Autodesk Inventor part; units mm, degrees
ref_plane "YZ Plane" through (0, 0, 0) normal (1, 0, 0) x (0, 1, 0)
ref_plane "XZ Plane" through (0, 0, 0) normal (0, 1, 0) x (-1, 0, 0)
ref_plane "XY Plane" through (0, 0, 0) normal (0, 0, 1) x (1, 0, 0)
sketch "스케치1" plane through (0, 0, 0) normal (0, 0, 1) x (1, 0, 0)
  line L0 (50, 0) -> (50, 28)
  line L1 (-50, 28) -> (-50, 0)
  line L2 (32, 28) -> (32, 38)
  line L3 (-32, 38) -> (-32, 28)
  line L4 (-40, 38) -> (-40, 60)
  line L5 (40, 60) -> (40, 38)
  line L6 (-35.94, 60) -> (-3.94, 28)
  line L7 (3.94, 28) -> (35.94, 60)
  line L8 (-40, 60) -> (-35.94, 60)
  line L9 (35.94, 60) -> (40, 60)
  line L10 (3.94, 28) -> (4.06, 28)
  line L11 (4.06, 28) -> (4.06, 24.06)
  line L12 (4.06, 24.06) -> (-3.94, 24.06)
  line L13 (-3.94, 24.06) -> (-3.94, 28)
  line L14 (-32, 28) -> (-3.94, 28)
  line L15 (3.94, 28) -> (32, 28)
  line L16 (50, 28) -> (3.94, 28)
  line L17 (-3.94, 28) -> (-50, 28)
  line L18 (32, 38) -> (13.94, 38)
  line L19 (-13.94, 38) -> (-32, 38)
  line L20 (40, 38) -> (13.94, 38)
  line L21 (-13.94, 38) -> (-40, 38)
  line L22 (4.06, 0) -> (5, 0)
  line L23 (5, 0) -> (5, 5.8283)
  line L24 (5, 5.8283) -> (-5, 5.8283)
  line L25 (-5, 5.8283) -> (-5, 0)
  line L26 (-50, 0) -> (-5, 0)
  line L27 (5, 0) -> (50, 0)
  point P0 (0, 0)
  point P1 (0, 0)
  dimension "d0" = 100
  dimension "d1" = 28
  dimension "d2" = 50
  dimension "d3" = 64
  dimension "d4" = 32
  dimension "d5" = 10
  dimension "d6" = 80
  dimension "d8" = 40
  dimension "d11" = 90
  dimension "d12" = 80
  dimension "d13" = 4.06
  dimension "d14" = 4.06
  dimension "d15" = 8
  dimension "d16" = 10
  dimension "d17" = 5
extrude "돌출1" add sketch "스케치1" along normal mid plane 48
sketch "스케치2" plane through (50, 0, 24) normal (1, 0, 0) x (0, 0, -1)
  line L0 (48, 0) -> (0, 0)
  line L1 (48, 5.8283) -> (0, 5.8283)
  line L2 (19.5, 0) -> (28.5, 0)
  line L3 (28.5, 0) -> (28.5, 5.8283)
  line L4 (28.5, 5.8283) -> (19.5, 5.8283)
  line L5 (19.5, 5.8283) -> (19.5, 0)
  point P0 (24, 0)
  dimension "d20" = 9
  dimension "d21" = 4.5
extrude "돌출2" cut sketch "스케치2" against normal through all
sketch "스케치3" plane through (-5, 5.8283, 24) normal (0, -1, 0) x (1, 0, 0)
  circle A0 centre (5, -24) radius 4.5
  dimension "d24" = 9
extrude "돌출3" cut sketch "스케치3" against normal through all
properties part number "부품1"
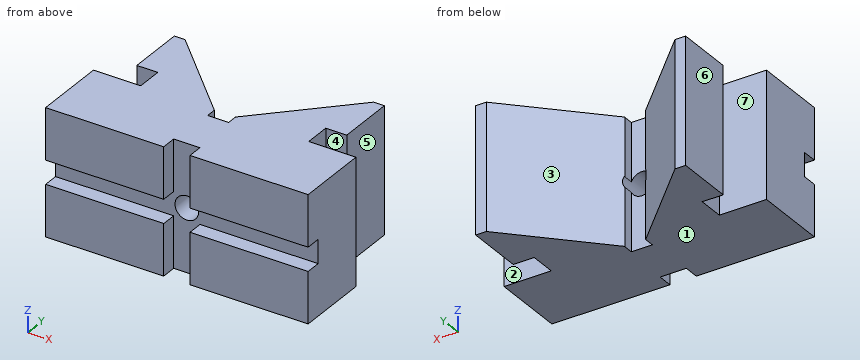
Here's how the part is built. I have some questions about the finished solid (model axes, mm). Face numbers are marked on the shaded views. A direction names the side the tool comes from. Round coordinates to 2 decimals unless told otherwise and drop trailing zeros. Write each loop counter-clockwise with the first axis right and the second up, starting at its lowest first coordinate (ties: lowest second). Pieces come first, ordered by that corner, then holes.
Q1. Which directions (+Z, -Z, +X, -X, +Y, -Y) give clear straight access to the entire face, cutting with the end or side of a thin tool? Please do the marked faces 5, 6 and 7.
Q2. Will these pins go through, and if not, where does the flat tip stop? P1, Ø11.5, axis at x = 0, z = 0, coming from the -Y side; P2, Ø6, axis at x = -13.5, z = 18, coming from the +Y side; P3, Ø5, axis at y = 34.5, z = -5.5, coming from the -X side.
Q3. If we section it at B-B on z = 0: Write out the boundary of the cut face in (x, y), plus the area to 3 significant figures.
Q4. Please list where these lines run through material, in increasing order: probe 1 along X at (y, z) = (21, 0); probe 2 along Z at (x, y) = (0, 11.5); probe 3 along X at (y, z) = (4.5, 21).
Q5. If we section it at A-A on y = 48: Write out the boundary of the cut face in (x, z), plus the area to 3 significant figures.
Q6. If we section it at C-C on x = -34: Write out the boundary of the cut face in (y, z), plus the area to 3 significant figures.
Q7. If we section it at D-D on x = 17.5: Write out the boundary of the cut face in (y, z), plus the area to 3 significant figures.
Q8. If we mould it in two halves opening along Y, with no side actions, what happens to the marked faces 1, 2, 3 and 4? For each: +Y half, -Y half, draft (parallel to the pull), parting line (faces both ways), or undercut.
Answer below:
1. face 5: +Z, -Z, +X, +Y
1. face 6: +Z, -Z, -X, +Y
1. face 7: +Z, -Z, -X
2. P1: stops at y = 5.83
2. P2: stops at y = 40.56
2. P3: stops at x = -32
3. outline: (-50, 5.83) - (-4.5, 5.83) - (-4.5, 28.56) - (-35.94, 60) - (-40, 60) - (-40, 38) - (-32, 38) - (-32, 28) - (-50, 28) - close; (4.5, 5.83) - (50, 5.83) - (50, 28) - (32, 28) - (32, 38) - (40, 38) - (40, 60) - (35.94, 60) - (4.5, 28.56) - close
3. area: 3,140 mm2
4. probe 1: x = -50 to -4.5, 4.5 to 50
4. probe 2: z = -24 to -4.5, 4.5 to 24
4. probe 3: x = -50 to -5, 5 to 50
5. outline: (-40, -24) - (-23.94, -24) - (-23.94, 24) - (-40, 24) - close; (23.94, -24) - (40, -24) - (40, 24) - (23.94, 24) - close
5. area: 1,540 mm2
6. outline: (0, -24) - (28, -24) - (28, 24) - (0, 24) - (0, 4.5) - (5.83, 4.5) - (5.83, -4.5) - (0, -4.5) - close; (38, -24) - (58.06, -24) - (58.06, 24) - (38, 24) - close
6. area: 2,250 mm2
7. outline: (0, -24) - (41.56, -24) - (41.56, 24) - (0, 24) - (0, 4.5) - (5.83, 4.5) - (5.83, -4.5) - (0, -4.5) - close
7. area: 1,940 mm2
8. face 1: draft
8. face 2: undercut
8. face 3: +Y half
8. face 4: undercut
